For this review, use the dimensioned drawing (mm, ordinates from the lowest corner) and the shaded views. A direction names the side the tool comes from. Give positions to 0.01 mm unless a question says otherwise; leave off trailing zeros. Write each loop counter-clockwise with the first axis right and the second up, starting at its lowest first coordinate (ties: lowest second). Pieces come first, ordered by that corner, then holes. Notation, with made-up numbers: M 56,50 L 61,50 A11 cw 61,69 Z; hole C 26,54 d2. An arc over 180 degrees is marked long. One line per item, written item: value. Start each with the question number.
Item 1: Consider section B-B, the plane y = 2.8. Write out the cut boundary in (x, z).
Item 2: Clearance check with flat-ended pins moving along their axes: pin 1 Ø5 at (x, z) = (71, 4.5) entering from -Y; pin 2 Ø1.9 at (x, y) = (84, 2.8) entering from +Z; pin 3 Ø1.7 at (x, y) = (72.5, 4) entering from +Z. State where each tip first meets the part, or that it passes through.
Item 3: Consider section A-A, the plane x = 6. Write out the cut boundary in (y, z), and give its area (3 significant figures).
Item 4: Tool access review of the marked faces 1 and 2: name each direction out of +Z, -Z, +X, -X, +Y, -Y from which nothing blocks a thin tool from reaching the whole face with its end or side.
Item 5: To check wall thickness, follow probe 1 along Z at (x, y) = (92, 6.75); probe 2 along X at (y, z) = (4, 1); probe 3 along Y at (x, z) = (14, 1). State the ranges of each line that lie inside material, in increasing order.
Item 6: Consider section C-C, the plane z = 6. Write out the cut boundary in (x, y).
Item 7: Consider section D-D, the plane x = 17. Write out the cut boundary in (y, z), and give its area (3 significant figures).
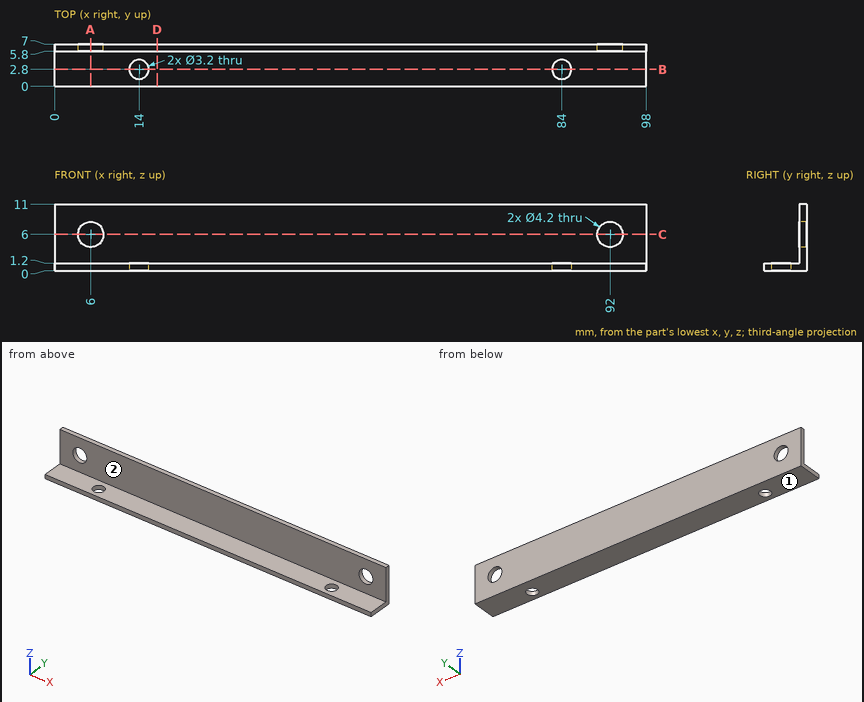
Model answer:
1. outline: M 0,0 L 12.4,0 L 12.4,1.2 L 0,1.2 Z; M 15.6,0 L 82.4,0 L 82.4,1.2 L 15.6,1.2 Z; M 85.6,0 L 98,0 L 98,1.2 L 85.6,1.2 Z
2. pin 1: stops at y = 5.8
2. pin 2: passes through
2. pin 3: stops at z = 1.2
3. outline: M 0,0 L 7,0 L 7,3.9 L 5.8,3.9 L 5.8,1.2 L 0,1.2 Z; M 5.8,8.1 L 7,8.1 L 7,11 L 5.8,11 Z
3. area: 15.1 mm2
4. face 1: -Z, +X, -X, +Y, -Y
4. face 2: +Z, +X, -X, -Y
5. probe 1: z = 0 to 3.9, 8.1 to 11
5. probe 2: x = 0 to 12.94, 15.06 to 82.94, 85.06 to 98
5. probe 3: y = 0 to 1.2, 4.4 to 7
6. outline: M 0,5.8 L 3.9,5.8 L 3.9,7 L 0,7 Z; M 8.1,5.8 L 89.9,5.8 L 89.9,7 L 8.1,7 Z; M 94.1,5.8 L 98,5.8 L 98,7 L 94.1,7 Z
7. outline: M 0,0 L 7,0 L 7,11 L 5.8,11 L 5.8,1.2 L 0,1.2 Z
7. area: 20.2 mm2
